Geometry: final body of the model. Coordinates: model frame, mm. Face numbers are marked on the shaded views. A direction names the side the tool comes from. Round coordinates to 2 decimals unless told otherwise and drop trailing zeros. Write each loop counter-clockwise with the first axis right and the second up, starting at its lowest first coordinate (ties: lowest second). Pieces come first, ordered by that corner, then holes. Notation, with made-up numbers: (-16.75, 54) -> (12.25, 54) arc R25 ccw to (12.25, 85) -> close; hole circle Ø4 at (71, 10). An arc over 180 degrees is marked (long way). Use one line per item in the form item = value. Start each with the question number.
1. Cut plane D-D, the plane z = 2. Return the cut outline in (x, y), plus the area to 3 significant figures.
2. Draft query along Y for the marked faces 1, 2 and 3. Return one class per face: pulls with the +Y half, pulls with the -Y half, needs draft (parallel to the pull), parting line crosses it, or undercut.
3. Pin query (flat end, axial travel): pin 1 Ø2.5 at (x, y) = (0, 0) entering from +Z; pin 2 Ø3 at (x, z) = (-10.5, 6) entering from +Y; pin 3 Ø1 at (x, z) = (-14.5, 9) entering from -Y. Return the tip coordinate at first contact, or that it passes through.
4. Cut plane B-B, the plane x = 0. Return the cut outline in (y, z).
5. Reachability of the marked faces 4 and 5 from +Z, -Z, +X, -X, +Y, -Y: full face, straight path, thin tool, end or side. Return the list, or none.
6. Cut plane A-A, the plane y = 0. Return the cut outline in (x, z).
7. Cut plane C-C, the plane z = 14. Return the cut outline in (x, y), plus the area to 3 significant figures.
8. Line query: L1, parallel to Z at x = 0.5, y = 9; L2, parallel to Y at x = 0, z = 14.5; L3, parallel to X at y = -4.5, z = 13. Output: solid intervals per line, ascending.
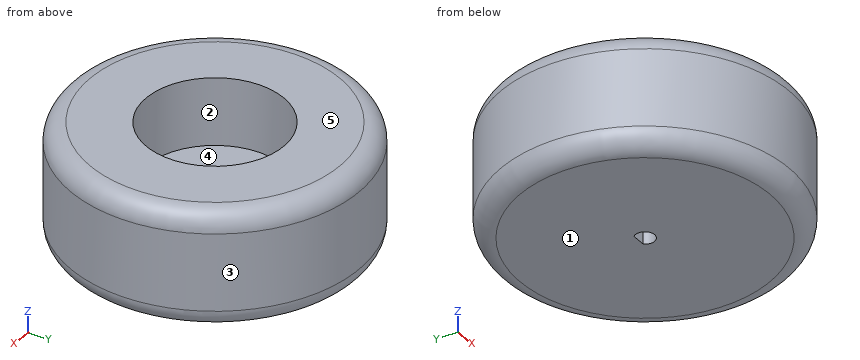
```python
from build123d import *

# Parameters (mm, degrees)
CUT_EXTRUDE1_DEPTH = 37.558172882


with BuildPart() as part:
    # Sketch1 → Revolve1 (revolve)
    with BuildSketch(Plane(origin=(0, 0, 0), x_dir=(1, 0, 0), z_dir=(0, 1, 0)), mode=Mode.PRIVATE) as revolve1_sk:
        with BuildLine():
            Line((0, 0), (19.5, 0))
            ThreePointArc((19.5, 0), (21.621320344, -0.878679656), (22.5, -3))
            Line((22.5, -3), (22.5, -15))
            ThreePointArc((22.5, -15), (21.621320344, -17.121320344), (19.5, -18))
            Line((19.5, -18), (10.75, -18))
            Line((10.75, -18), (10.75, -7.5))
            Line((10.75, -7.5), (0, -7.5))
            Line((0, -7.5), (0, 0))
        make_face()
    revolve(revolve1_sk.sketch.rotate(Axis((0, 0, -41.848991251), (0, 0, 1)), 180), axis=Axis((0, 0, -41.848991251), (0, 0, 1)))

    # Sketch2 → Cut-Extrude1 (cut, through all)
    with BuildSketch(Plane.XY):
        with BuildLine():
            Line((-1.118033989, 1), (1.118033989, 1))
            ThreePointArc((1.118033989, 1), (0, -1.5), (-1.118033989, 1))
        make_face()
    extrude(amount=CUT_EXTRUDE1_DEPTH, mode=Mode.SUBTRACT)


solid = part.part
```
Outcome:
q1.outline = circle Ø44.66 at (0, 0); hole (-1.12, 1) arc R1.5 ccw (long way) to (1.12, 1) -> close
q1.area = 1,560 mm^2
q2.face_1 = needs draft
q2.face_2 = undercut
q2.face_3 = parting line crosses it
q3.pin_1 = 7.5
q3.pin_2 = 20.62
q3.pin_3 = -17.61
q4.outline = (-22.5, 3) arc R3 ccw to (-19.5, 0) -> (-1.5, 0) -> (-1.5, 7.5) -> (-10.75, 7.5) -> (-10.75, 18) -> (-19.5, 18) arc R3 ccw to (-22.5, 15) -> close; (1, 0) -> (19.5, 0) arc R3 ccw to (22.5, 3) -> (22.5, 15) arc R3 ccw to (19.5, 18) -> (10.75, 18) -> (10.75, 7.5) -> (1, 7.5) -> close
q5.face_4 = +Z
q5.face_5 = +Z, +X, -X, +Y, -Y
q6.outline = (-22.5, 3) arc R3 ccw to (-19.5, 0) -> (-1.5, 0) -> (-1.5, 7.5) -> (-10.75, 7.5) -> (-10.75, 18) -> (-19.5, 18) arc R3 ccw to (-22.5, 15) -> close; (1.5, 0) -> (19.5, 0) arc R3 ccw to (22.5, 3) -> (22.5, 15) arc R3 ccw to (19.5, 18) -> (10.75, 18) -> (10.75, 7.5) -> (1.5, 7.5) -> close
q7.outline = circle Ø45 at (0, 0); hole circle Ø21.5 at (0, 0)
q7.area = 1,230 mm^2
q8.L1 = 0 to 7.5
q8.L2 = -22.5 to -10.75, 10.75 to 22.5
q8.L3 = -22.05 to -9.76, 9.76 to 22.05
